from build123d import *

# Parameters (mm, degrees)
SKETCH1_W           = 58.42
SKETCH1_H           = 31.75
BOSS_EXTRUDE1_DEPTH = 2.54
FILLET1_R           = 2.54
SKETCH4_R           = 5.08
BOSS_EXTRUDE3_DEPTH = 15.875
SKETCH5_R           = 5.08
BOSS_EXTRUDE4_DEPTH = 10.16
SKETCH6_R           = 3.556
CUT_EXTRUDE2_DEPTH  = 32.75
SKETCH9_W           = 13.97
SKETCH9_H           = 3.81
CUT_EXTRUDE4_DEPTH  = 1.27
SKETCH10_W          = 2.54
SKETCH10_H          = 2.54
SKETCH10_W_2        = 20.32
SKETCH10_H_2        = 3.81
CUT_EXTRUDE6_DEPTH  = 12.176
SKETCH11_W          = 71.12
SKETCH11_H          = 2.54
BOSS_EXTRUDE5_DEPTH = 15.875
SKETCH12_W          = 71.12
SKETCH12_H          = 2.54
BOSS_EXTRUDE6_DEPTH = 6.35
FILLET2_R           = 2.54
SKETCH13_W          = 2.54
SKETCH13_H          = 2.54
CUT_EXTRUDE7_DEPTH  = 2.54
SKETCH14_W          = 2.54
SKETCH14_H          = 2.54
SKETCH14_W_2        = 2.546026668
CUT_EXTRUDE8_DEPTH  = 13.192


with BuildPart() as part:
    # Sketch1 → Boss-Extrude1 (new body)
    with BuildSketch(Plane(origin=(0, 0, 0), x_dir=(1, 0, 0), z_dir=(0, 1, 0))):
        Rectangle(SKETCH1_W, SKETCH1_H)
    extrude(amount=BOSS_EXTRUDE1_DEPTH)

    # Fillet1
    fillet1_edges = [part.edges().sort_by_distance(p)[0] for p in [
        (29.21, 1.27, 15.875),
        (-29.21, 1.27, 15.875),
        (-29.21, 1.27, -15.875),
        (29.21, 1.27, -15.875),
    ]]
    fillet(fillet1_edges, radius=FILLET1_R)

    # Sketch4 → Boss-Extrude3 (add)
    with BuildSketch(Plane.XY):
        with Locations((-19.05, 6.096)):
            Circle(SKETCH4_R)
        with Locations((19.05, 6.096)):
            Circle(SKETCH4_R)
    extrude(amount=BOSS_EXTRUDE3_DEPTH)

    # Sketch5 → Boss-Extrude4 (add)
    with BuildSketch(Plane(origin=(0, 0, 0), x_dir=(-1, 0, 0), z_dir=(0, 0, -1))):
        with Locations((-19.05, 6.096)):
            Circle(SKETCH5_R)
        with Locations((19.05, 6.096)):
            Circle(SKETCH5_R)
    extrude(amount=BOSS_EXTRUDE4_DEPTH)

    # Sketch6 → Cut-Extrude2 (cut, through all)
    with BuildSketch(Plane.XY.offset(15.875)):
        with Locations((-19.05, 6.096)):
            Circle(SKETCH6_R)
        with Locations((19.05, 6.096)):
            Circle(SKETCH6_R)
    extrude(amount=-CUT_EXTRUDE2_DEPTH, mode=Mode.SUBTRACT)

    # Sketch9 → Cut-Extrude4 (cut)
    with BuildSketch(Plane(origin=(0, 2.54, 0), x_dir=(1, 0, 0), z_dir=(0, 1, 0))):
        with Locations((-6.985, 13.97)):
            Rectangle(SKETCH9_W, SKETCH9_H)
        with Locations((6.985, 13.97)):
            Rectangle(SKETCH9_W, SKETCH9_H)
    extrude(amount=-CUT_EXTRUDE4_DEPTH, mode=Mode.SUBTRACT)

    # Sketch10 → Cut-Extrude6 (cut, through all)
    with BuildSketch(Plane(origin=(0, 0, 0), x_dir=(1, 0, 0), z_dir=(0, 1, 0))):
        with Locations((-27.94, 0)):
            Rectangle(SKETCH10_W, SKETCH10_H)
        with Locations((27.94, 0)):
            Rectangle(SKETCH10_W, SKETCH10_H)
        with Locations((0, 13.97)):
            Rectangle(SKETCH10_W_2, SKETCH10_H_2)
        with Locations((-8.89, -14.605)):
            Rectangle(SKETCH10_W, SKETCH10_H)
        with Locations((8.89, -14.605)):
            Rectangle(SKETCH10_W, SKETCH10_H)
    extrude(amount=CUT_EXTRUDE6_DEPTH, mode=Mode.SUBTRACT)

    # Sketch11 → Boss-Extrude5 (add)
    with BuildSketch(Plane.XY):
        with Locations((0, 10.922)):
            Rectangle(SKETCH11_W, SKETCH11_H)
    extrude(amount=BOSS_EXTRUDE5_DEPTH)

    # Sketch12 → Boss-Extrude6 (add)
    with BuildSketch(Plane(origin=(0, 0, 0), x_dir=(-1, 0, 0), z_dir=(0, 0, -1))):
        with Locations((0, 10.922)):
            Rectangle(SKETCH12_W, SKETCH12_H)
    extrude(amount=BOSS_EXTRUDE6_DEPTH)

    # Fillet2
    fillet2_edges = [part.edges().sort_by_distance(p)[0] for p in [
        (-35.56, 10.922, 15.875),
        (35.56, 10.922, 15.875),
        (-35.56, 10.922, -6.35),
        (35.56, 10.922, -6.35),
    ]]
    fillet(fillet2_edges, radius=FILLET2_R)

    # Sketch13 → Cut-Extrude7 (cut)
    with BuildSketch(Plane(origin=(0, 12.192, 0), x_dir=(1, 0, 0), z_dir=(0, 1, 0))):
        with Locations((-34.344972833, 0.003915147)):
            Rectangle(SKETCH13_W, SKETCH13_H)
        with Locations((8.89, -14.605)):
            Rectangle(SKETCH13_W, SKETCH13_H)
        with Locations((-8.89, -14.605)):
            Rectangle(SKETCH13_W, SKETCH13_H)
        with Locations((34.344972833, 0.003915147)):
            Rectangle(SKETCH13_W, SKETCH13_H)
        with Locations((8.89, 4.953)):
            Rectangle(SKETCH13_W, SKETCH13_H)
        with Locations((-8.89, 4.953)):
            Rectangle(SKETCH13_W, SKETCH13_H)
    extrude(amount=-CUT_EXTRUDE7_DEPTH, mode=Mode.SUBTRACT)

    # Sketch14 → Cut-Extrude8 (cut, through all)
    with BuildSketch(Plane(origin=(0, 0, -3.683), x_dir=(-1, 0, 0), z_dir=(0, 0, -1))):
        with Locations((8.89, 10.922)):
            Rectangle(SKETCH14_W, SKETCH14_H)
        with Locations((-8.893013334, 10.922)):
            Rectangle(SKETCH14_W_2, SKETCH14_H)
    extrude(amount=CUT_EXTRUDE8_DEPTH, mode=Mode.SUBTRACT)


solid = part.part
Model file for the job. Use its own axes, mm. A direction names the side the tool comes from. Give positions to 0.01 mm unless a question says otherwise; leave off trailing zeros. Loops run counter-clockwise (first coordinate to the right, second up) from the corner with the lowest first, then second, coordinate; pieces in that order, holes last.
1) Saw through at A-A (x = -1). Write the cut outline in (y, z) (3 decimals).
2) Flat gauge pins, fed straight in: pin 1 Ø2.5 at (x, y) = (34.5, 11) entering from +Z; pin 2 Ø2 at (y, z) = (8, 10.5) entering from -X; pin 3 Ø1.5 at (y, z) = (1.5, -3.5) entering from +X. Where does each tip first touch, or does it go through?
3) Wall check: line 1 (Y direction, x = 19, z = 9); line 2 (X direction, y = 3.75, z = 0); line 3 (X direction, y = 2.25, z = 9.5). Give the ranges that are in metal, low to high.
4) Saw through at D-D (z = 8.5). Write the cut outline in (x, y), plus the area to 3 significant figures.
5) Pull direction Y, two halves, no side cores. Call faces 4 (the flat face through (-9, 11, 13.335)), 5 (the flat face through (0, 9.652, 5)): +Y half, -Y half, draft (parallel to the pull), parting line (faces both ways), or undercut.
6) Saw through at C-C (y = 7.5). Write the cut outline in (x, z) (3 decimals), plus the area to 3 significant figures.
7) Saw through at B-B (z = -4.5). Write the cut outline in (x, y), plus the area to 3 significant figures.
8) Tool access for faces 1 (the flat face through (0, 11, -6.35)), 2 (the flat face through (9, 11, 13.335)), 3 (the flat face through (33.075, 11, 0)): list every direction of +Z, -Z, +X, -X, +Y, -Y with a clear straight run to the whole face (end or side of a thin tool).
Answer block:
1. outline: (0, -12.065) - (2.54, -12.065) - (2.54, 15.875) - (0, 15.875) - close; (9.652, -6.35) - (12.192, -6.35) - (12.192, 15.875) - (9.652, 15.875) - close
2. pin 1: stops at z = 15.86
2. pin 2: stops at x = -24.05
2. pin 3: stops at x = 29.21
3. line 1: y = 0 to 2.54, 9.65 to 12.19
3. line 2: x = -23.56 to -21.72, -16.38 to -14.54, 14.54 to 16.38, 21.72 to 23.56
3. line 3: x = -29.21 to 29.21
4. outline: (-35.56, 9.65) - (-22.68, 9.65) arc R5.08 ccw to (-22.68, 2.54) - (-29.21, 2.54) - (-29.21, 0) - (29.21, 0) - (29.21, 2.54) - (22.68, 2.54) arc R5.08 ccw to (22.68, 9.65) - (35.56, 9.65) - (35.56, 12.19) - (-35.56, 12.19) - close; hole circle Ø7.11 at (-19.05, 6.1); hole (-15.42, 2.54) - (15.42, 2.54) arc R5.08 cw to (15.42, 9.65) - (-15.42, 9.65) arc R5.08 cw to start; hole circle Ø7.11 at (19.05, 6.1)
4. area: 381 mm2
5. face 4: draft
5. face 5: undercut
6. outline: (-23.932, -10.16) - (-22.317, -10.16) - (-22.317, 15.875) - (-23.932, 15.875) - close; (-15.783, -10.16) - (-14.168, -10.16) - (-14.168, 15.875) - (-15.783, 15.875) - close; (14.168, -10.16) - (15.783, -10.16) - (15.783, 15.875) - (14.168, 15.875) - close; (22.317, -10.16) - (23.932, -10.16) - (23.932, 15.875) - (22.317, 15.875) - close
6. area: 168 mm2
7. outline: (-35.46, 9.65) - (-22.68, 9.65) arc R5.08 ccw to (-22.68, 2.54) - (-29.21, 2.54) - (-29.21, 0) - (29.21, 0) - (29.21, 2.54) - (22.68, 2.54) arc R5.08 ccw to (22.68, 9.65) - (35.46, 9.65) - (35.46, 12.19) - (10.17, 12.19) - (10.17, 9.65) - (15.42, 9.65) arc R5.08 ccw to (15.42, 2.54) - (-15.42, 2.54) arc R5.08 ccw to (-15.42, 9.65) - (-10.16, 9.65) - (-10.16, 12.19) - (-35.46, 12.19) - close; (-7.62, 9.65) - (7.62, 9.65) - (7.62, 12.19) - (-7.62, 12.19) - close; hole circle Ø7.11 at (-19.05, 6.1); hole circle Ø7.11 at (19.05, 6.1)
7. area: 368 mm2
8. face 1: -Z, +Y
8. face 2: +Z, +Y, -Y
8. face 3: +X, +Y, -Y
